Autodesk Inventor part; units mm, degrees
ref_plane "YZ Plane" through (0, 0, 0) normal (1, 0, 0) x (0, 1, 0)
ref_plane "XZ Plane" through (0, 0, 0) normal (0, 1, 0) x (-1, 0, 0)
ref_plane "XY Plane" through (0, 0, 0) normal (0, 0, 1) x (1, 0, 0)
sketch "Sketch1" plane through (0, 0, 0) normal (0, 0, 1) x (1, 0, 0)
  line L0 (0, 97.79) -> (0, -97.79)
  line L1 (-200.025, 0) -> (200.025, 0)
  line L2 (142.875, -69.85) -> (-142.875, -69.85)
  line L3 (-142.875, -69.85) -> (-142.875, 69.85)
  line L4 (-142.875, 69.85) -> (142.875, 69.85)
  line L5 (142.875, 69.85) -> (142.875, -69.85)
  line L6 (142.875, -69.85) -> (-142.875, 69.85) construction
  line L7 (-142.875, -69.85) -> (142.875, 69.85) construction
  line L8 (-136.525, -63.5) -> (136.525, -63.5) construction
  line L9 (136.525, -63.5) -> (136.525, 63.5) construction
  line L10 (136.525, 63.5) -> (-136.525, 63.5) construction
  line L11 (-136.525, 63.5) -> (-136.525, -63.5) construction
  line L12 (-136.525, -63.5) -> (136.525, 63.5) construction
  line L13 (136.525, -63.5) -> (-136.525, 63.5) construction
  line L14 (-100.965, -14.2875) -> (-114.935, -14.2875)
  line L15 (-114.935, -14.2875) -> (-114.935, 14.2875)
  line L16 (-114.935, 14.2875) -> (-100.965, 14.2875)
  line L17 (-100.965, 14.2875) -> (-100.965, -14.2875)
  line L18 (-100.965, -14.2875) -> (-114.935, 14.2875) construction
  line L19 (-114.935, -14.2875) -> (-100.965, 14.2875) construction
  circle A0 centre (44.45, 31.75) radius 10.795
  circle A1 centre (44.45, -31.75) radius 10.795
  circle A2 centre (95.25, 0) radius 11.303
  circle A3 centre (95.25, 0) radius 30 construction
  line L20 (-64.135, -14.2875) -> (-50.165, -14.2875)
  line L21 (-50.165, -14.2875) -> (-50.165, 14.2875)
  line L22 (-50.165, 14.2875) -> (-64.135, 14.2875)
  line L23 (-64.135, 14.2875) -> (-64.135, -14.2875)
  line L24 (-64.135, -14.2875) -> (-50.165, 14.2875) construction
  line L25 (-50.165, -14.2875) -> (-64.135, 14.2875) construction
  line L26 (7.9375, -6.985) -> (-20.6375, -6.985)
  line L27 (-20.6375, -6.985) -> (-20.6375, 6.985)
  line L28 (-20.6375, 6.985) -> (7.9375, 6.985)
  line L29 (7.9375, 6.985) -> (7.9375, -6.985)
  line L30 (7.9375, -6.985) -> (-20.6375, 6.985) construction
  line L31 (-20.6375, -6.985) -> (7.9375, 6.985) construction
  point P0 (0, 0)
  point P1 (-107.95, 0)
  point P2 (95.25, 14.732)
  point P3 (95.25, -14.732)
  point P4 (-19.05, 63.5)
  point P5 (-19.05, -63.5)
  point P6 (19.05, -63.5)
  point P7 (19.05, 63.5)
  point P8 (-57.15, 0)
  point P9 (-6.35, 0)
  dimension "d0" = 285.75
  dimension "d1" = 139.7
  dimension "d4" = 6.35
  dimension "d5" = 6.35
  dimension "d6" = 13.97
  dimension "d7" = 28.575
  dimension "d15" = 0
  dimension "d16" = 21.59
  dimension "d20" = 22.606
  dimension "d22" = 60
  dimension "d33" = 47.625
  dimension "d34" = 14.732
  dimension "d35" = 14.732
  dimension "d43" = 34.925
  dimension "d44" = 31.75
  dimension "d45" = 31.75
  dimension "d46" = 152.4
  dimension "d47" = 50.8
  dimension "d48" = 19.05
  dimension "d49" = 19.05
  dimension "d50" = 50.8
  dimension "d51" = 50.8
extrude "Extrusion1" add sketch "Sketch1" along normal blind 3.175 contours L4 L5 L1 A2 L29 L28 L0 | L0 L28 L27 L1 L21 L22 L23 L17 L16 L15 L3 L4 | L1 L15 L14 L17 L23 L20 L21 L27 L26 L0 L2 L3 | L5 L2 L0 L26 L29 L1 A2
hole "Hole1" at (-136.525, 63.5, 0) at (-136.525, -63.5, 0) at (136.525, 63.5, 0) at (136.525, -63.5, 0) at (19.05, -63.5, 0) at (-19.05, 63.5, 0) at (19.05, 63.5, 0) at (-19.05, -63.5, 0) direction (0, 0, 1) diameter 5.08 end through all
fillet "Fillet1" radius 6.35 4 edges at (142.875, -69.85, 1.5875) (142.875, 69.85, 1.5875) (-142.875, -69.85, 1.5875) (-142.875, 69.85, 1.5875)
hole "Hole2" at (95.25, 14.732, 0) at (95.25, -14.732, 0) direction (0, 0, 1) diameter 3.1242 end through all
The listing builds one solid part. Answer for the finished solid, in the listing's coordinates (mm). Round coordinates to 2 decimals unless told otherwise and drop trailing zeros. Order: outer loops, then holes, each group sorted by start corner. A loop starts at its lowest first (then second) coordinate and runs counter-clockwise, first axis right, second up. Notation, with made-up numbers: M 78.5,-36 L 86.5,-36 A6 cw 86.5,-28 Z; hole C 72,-6 d8. An arc over 180 degrees is marked long. Answer in a Markdown table with one row per item. Add a question column.
1) A flat-ended cylindrical pin translates along its axis: pin 1 Ø3.5 at (x, y) = (95.25, -14.732) entering from -Z. Find the tip coordinate at first contact, or state that the pin passes through.
2) Consider line 1 along X through (y, z) = (-63.5, 1.55) (3 decimals); line 2 along Y through (x, z) = (19.05, 1); line 3 along X through (y, z) = (-64, 1.25). Determine where each line is inside the solid, lowest interval first. Write a range as from..to.
3) The part is cut by section C-C on z = 1.1. Count the separate pieces of the cut face and the enclosed holes in it, plus the area to 3 significant figures.
4) The part is cut by section D-D on y = -31.75. Determine the outline of the cut face in (x, z) (3 decimals).
5) The part is cut by section B-B on y = 0. Determine the outline of the cut face in (x, z) (1 decimal).
Findings below:
| question | item | result |
|---|---|---|
| 1 | pin 1 | stops at z = 0 |
| 2 | line 1 | x = -142.875..-139.065, -133.985..-21.59, -16.51..16.51, 21.59..133.985, 139.065..142.875 |
| 2 | line 2 | y = -69.85..-66.04, -60.96..60.96, 66.04..69.85 |
| 2 | line 3 | x = -142.86..-139.02, -134.03..-21.54, -16.56..16.56, 21.54..134.03, 139.02..142.86 |
| 3 | separate pieces | 1 |
| 3 | enclosed holes | 16 |
| 3 | area | 37,400 mm² |
| 4 | outline | M -142.875,0 L 33.655,0 L 33.655,3.175 L -142.875,3.175 Z; M 55.245,0 L 142.875,0 L 142.875,3.175 L 55.245,3.175 Z |
| 5 | outline | M -142.9,0 L -114.9,0 L -114.9,3.2 L -142.9,3.2 Z; M -101,0 L -64.1,0 L -64.1,3.2 L -101,3.2 Z; M -50.2,0 L -20.6,0 L -20.6,3.2 L -50.2,3.2 Z; M 7.9,0 L 83.9,0 L 83.9,3.2 L 7.9,3.2 Z; M 106.6,0 L 142.9,0 L 142.9,3.2 L 106.6,3.2 Z |
